Here's how the part is built. I have some questions about the finished solid (model axes, mm). Round coordinates to 2 decimals unless told otherwise and drop trailing zeros. Order: outer loops, then holes, each group sorted by start corner. A loop starts at its lowest first (then second) coordinate and runs counter-clockwise, first axis right, second up. Notation, with made-up numbers: (-18, -29) - (41, -29) arc R4 cw to (41, -23) - close; hole circle Ø8 at (68, -40). An arc over 180 degrees is marked (long way). One line per item, written item: value.
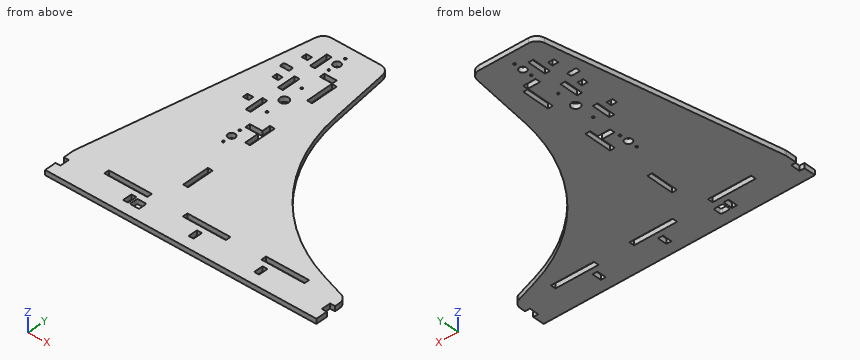
from build123d import *

# Parameters (mm, degrees)
MODEL_R             = 3.915
MODEL_R_2           = 1.2
MODEL_R_3           = 4.75
MODEL_R_4           = 3.95
MODEL_W             = 46.666
MODEL_H             = 5.5
MODEL_W_2           = 5.35
MODEL_H_2           = 10
MODEL_W_3           = 6.35
MODEL_H_3           = 5.35
MODEL_H_4           = 20
MODEL_H_5           = 29.666
MODEL_W_4           = 13.5
BOSS_EXTRUDE1_DEPTH = 5.35


with BuildPart() as part:
    # Model → Boss-Extrude1 (new body)
    with BuildSketch(Plane.XY):
        with BuildLine():
            Line((-147, 22.5), (-147, 33.91))
            ThreePointArc((-147, 33.91), (-146.957472748, 34.831268946), (-146.830252706, 35.744702086))
            Line((-146.830252706, 35.744702086), (-102.020252706, 275.834702086))
            ThreePointArc((-102.020252706, 275.834702086), (-98.579560984, 281.692432023), (-92.19, 284))
            Line((-92.19, 284), (-38.8, 284))
            ThreePointArc((-38.8, 284), (-32.222459634, 281.532327843), (-28.891161913, 275.347192548))
            Line((-28.891161913, 275.347192548), (-19.790761745, 208.412149045))
            ThreePointArc((-19.790761745, 208.412149045), (24.403039643, 107.726661994), (115.140729145, 45.619246274))
            Line((115.140729145, 45.619246274), (140.162263543, 37.27877618))
            ThreePointArc((140.162263543, 37.27877618), (145.112417501, 33.639047376), (147, 27.791938494))
            Line((147, 27.791938494), (147, 22.5))
            Line((147, 22.5), (141.65, 22.5))
            Line((141.65, 22.5), (141.65, 12.5))
            Line((141.65, 12.5), (147, 12.5))
            Line((147, 12.5), (147, 0))
            Line((147, 0), (-147, 0))
            Line((-147, 0), (-147, 12.5))
            Line((-147, 12.5), (-141.65, 12.5))
            Line((-141.65, 12.5), (-141.65, 22.5))
            Line((-141.65, 22.5), (-147, 22.5))
        make_face()
        with Locations((-65.5, 261)):
            Circle(MODEL_R, mode=Mode.SUBTRACT)
        with Locations((-65.5, 271)):
            Circle(MODEL_R_2, mode=Mode.SUBTRACT)
        with Locations((-65.5, 251)):
            Circle(MODEL_R_2, mode=Mode.SUBTRACT)
        with Locations((-65.5, 197.5)):
            Circle(MODEL_R_3, mode=Mode.SUBTRACT)
        with Locations((-65.5, 218.5)):
            Circle(MODEL_R_2, mode=Mode.SUBTRACT)
        with Locations((-65.5, 176.5)):
            Circle(MODEL_R_2, mode=Mode.SUBTRACT)
        with Locations((-65.5, 134.001)):
            Circle(MODEL_R_4, mode=Mode.SUBTRACT)
        with Locations((-65.5, 144.001)):
            Circle(MODEL_R_2, mode=Mode.SUBTRACT)
        with Locations((-65.5, 124.001)):
            Circle(MODEL_R_2, mode=Mode.SUBTRACT)
        with Locations((-0.001, 31.25)):
            Rectangle(MODEL_W, MODEL_H, mode=Mode.SUBTRACT)
        with Locations((-85.167, 31.25)):
            Rectangle(MODEL_W, MODEL_H, mode=Mode.SUBTRACT)
        with Locations((85.165, 31.25)):
            Rectangle(MODEL_W, MODEL_H, mode=Mode.SUBTRACT)
        with Locations((0.005, 17.5)):
            Rectangle(MODEL_W_2, MODEL_H_2, mode=Mode.SUBTRACT)
        with Locations((-71.075, 17.5)):
            Rectangle(MODEL_W_2, MODEL_H_2, mode=Mode.SUBTRACT)
        with Locations((71.085, 17.5)):
            Rectangle(MODEL_W_2, MODEL_H_2, mode=Mode.SUBTRACT)
        with Locations((-90.025, 216.5)):
            Rectangle(MODEL_W_3, MODEL_H_3, mode=Mode.SUBTRACT)
        with BuildLine():
            Line((-64.85, 21.33), (-57.85, 21.33))
            ThreePointArc((-57.85, 21.33), (-56.789339828, 20.890660172), (-56.35, 19.83))
            Line((-56.35, 19.83), (-56.35, 13.83))
            ThreePointArc((-56.35, 13.83), (-56.789339828, 12.769339828), (-57.85, 12.33))
            Line((-57.85, 12.33), (-64.85, 12.33))
            ThreePointArc((-64.85, 12.33), (-65.910660172, 12.769339828), (-66.35, 13.83))
            Line((-66.35, 13.83), (-66.35, 19.83))
            ThreePointArc((-66.35, 19.83), (-65.910660172, 20.890660172), (-64.85, 21.33))
        make_face(mode=Mode.SUBTRACT)
        with Locations((-90.025, 251.85)):
            Rectangle(MODEL_W_3, MODEL_H_3, mode=Mode.SUBTRACT)
        with Locations((-90.025, 181.15)):
            Rectangle(MODEL_W_3, MODEL_H_3, mode=Mode.SUBTRACT)
        with Locations((-77.825, 216.5)):
            Rectangle(MODEL_W_2, MODEL_H_4, mode=Mode.SUBTRACT)
        with Locations((-77.825, 255.25)):
            Rectangle(MODEL_W_2, MODEL_H_4, mode=Mode.SUBTRACT)
        with Locations((-77.825, 177.75)):
            Rectangle(MODEL_W_2, MODEL_H_4, mode=Mode.SUBTRACT)
        Polygon((-51.4, 164.334), (-46.05, 164.334), (-46.05, 134.668), (-51.4, 134.668), (-51.4, 150.001), (-64.9, 150.001), (-64.9, 155.351), (-51.4, 155.351), align=None, mode=Mode.SUBTRACT)
        with BuildLine():
            Line((-89.595, 228.801), (-97.595, 228.801))
            ThreePointArc((-97.595, 228.801), (-98.302106781, 229.093893219), (-98.595, 229.801))
            Line((-98.595, 229.801), (-98.595, 232.801))
            ThreePointArc((-98.595, 232.801), (-98.302106781, 233.508106781), (-97.595, 233.801))
            Line((-97.595, 233.801), (-89.595, 233.801))
            ThreePointArc((-89.595, 233.801), (-88.887893219, 233.508106781), (-88.595, 232.801))
            Line((-88.595, 232.801), (-88.595, 229.801))
            ThreePointArc((-88.595, 229.801), (-88.887893219, 229.093893219), (-89.595, 228.801))
        make_face(mode=Mode.SUBTRACT)
        with Locations((-48.725, 224.167)):
            Rectangle(MODEL_W_2, MODEL_H_5, mode=Mode.SUBTRACT)
        with Locations((-48.725, 74.835)):
            Rectangle(MODEL_W_2, MODEL_H_5, mode=Mode.SUBTRACT)
        with Locations((-58.15, 242.325)):
            Rectangle(MODEL_W_4, MODEL_H_3, mode=Mode.SUBTRACT)
    extrude(amount=BOSS_EXTRUDE1_DEPTH)


solid = part.part
Q1. If I drill on line 1 along Y through (x, z) = (-70.5, 1.3); line 2 along X through (y, z) = (229, 3.45); line 3 along X through (y, z) = (176.5, 3.8), over which ranges is the centre line in solid material (lowest first)?
Results list:
line 1: 0 to 12.5, 22.5 to 28.5, 34 to 284
line 2: -110.76 to -98.19, -89 to -51.4, -46.05 to -22.59
line 3: -120.56 to -80.5, -75.15 to -66.7, -64.3 to -12.76
Q2. If we section it at A-A, the plane x = 81.5: Please give me the cut outline in (y, z), then the cut area to 3 significant figures.
Results list:
outline: (0, 0) - (28.5, 0) - (28.5, 5.35) - (0, 5.35) - close; (34, 0) - (60.39, 0) - (60.39, 5.35) - (34, 5.35) - close
area: 294 mm²
Q3. If we section it at C-C, the plane z = 1.3: Give the number of separate pieces and of enclosed holes in the cut face, then the cut area to 3 significant figures.
Results list:
separate pieces: 1
enclosed holes: 27
area: 41,600 mm²
Q4. Will these pins go through, and if not, where does the flat tip stop? pin 1 (6.5 mm diameter, centred on x = -65.5, y = 134.001, fed in from +Z); pin 2 (2.5 mm diameter, centred on y = 32.5, z = 3, fed in from +X); pin 3 (1.6 mm diameter, centred on y = 18.5, z = 2, fed in from +X); pin 4 (1.6 mm diameter, centred on x = 143.5, z = 2, fed in from +Y).
Results list:
pin 1: through
pin 2: x = 146.38
pin 3: x = 141.65
pin 4: y = 36.01
Q5. If we section it at D-D, the plane x = 38.5: Please give me the cut outline in (y, z).
Results list:
outline: (0, 0) - (92.42, 0) - (92.42, 5.35) - (0, 5.35) - close
Q6. If we section it at B-B, the plane y = 261: Please give me the cut outline in (x, z) (3 decimals).
Results list:
outline: (-104.789, 0) - (-80.5, 0) - (-80.5, 5.35) - (-104.789, 5.35) - close; (-75.15, 0) - (-69.415, 0) - (-69.415, 5.35) - (-75.15, 5.35) - close; (-61.585, 0) - (-26.941, 0) - (-26.941, 5.35) - (-61.585, 5.35) - close
